The listing builds one solid part. Answer for the finished solid, in the listing's coordinates (mm). Face numbers are marked on the shaded views. A direction names the side the tool comes from. Round coordinates to 2 decimals unless told otherwise and drop trailing zeros. Order: outer loops, then holes, each group sorted by start corner. A loop starts at its lowest first (then second) coordinate and runs counter-clockwise, first axis right, second up. Notation, with made-up numbers: (1, 10.5) -> (9, 10.5) arc R20 ccw to (9, 34.5) -> close; hole circle Ø9 at (80.25, 6). An arc over 180 degrees is marked (long way). Answer in a Markdown table with one row per item. Add a question column.
```python
from build123d import *

# Parameters (mm, degrees)
SK_CBORE_R      = 5
BD_CBORE_DEPTH  = 5
SK_THREAD_R     = 2.5
BD_THREAD_DEPTH = 20
CF_CBORE_SIZE   = 0.5


with BuildPart() as part:
    # SK_CBORE → BD_CBORE (new body)
    with BuildSketch(Plane(origin=(0, 0, 0), x_dir=(0, 0, -1), z_dir=(0, 1, 0))):
        Circle(SK_CBORE_R)
    extrude(amount=BD_CBORE_DEPTH)

    # SK_THREAD → BD_THREAD (add)
    with BuildSketch(Plane.XZ):
        Circle(SK_THREAD_R)
    extrude(amount=BD_THREAD_DEPTH)

    # CF_CBORE
    cf_cbore_edges = [part.edges().sort_by_distance(p)[0] for p in [
        (0, 5, 5),
    ]]
    chamfer(cf_cbore_edges, length=CF_CBORE_SIZE)


solid = part.part
```
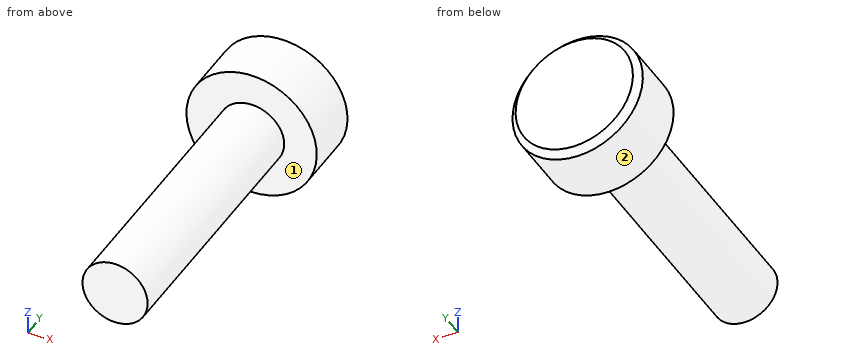
Item 1: Find the intervals of material crossed by probe 1 along Y at (x, z) = (3, 3); probe 2 along X at (y, z) = (-10, -1.5); probe 3 along Z at (x, y) = (2.5, 3.5), in increasing order. Write a range as [from, to].
Item 2: The part is cut by section A-A, the plane x = 0. Give the vertices of the cut face in (y, z), and give its area (3 significant figures).
Item 3: The part is cut by section C-C, the plane y = -4.5. Give the vertices of the cut face in (x, z), and give its area (3 significant figures).
Item 4: Flat-ended cylindrical pins translate along their axes: P1, Ø5, axis at x = -2.5, y = -9.5, coming from the +Z side; P2, Ø2, axis at y = -9.5, z = -1, coming from the +X side. Find the tip coordinate at first contact, or state that the pin passes through.
Item 5: A tool of negligible diameter and unlimited length cuts with its end or side. For the marked faces 1 and 2, from which of +Z, -Z, +X, -X, +Y, -Y can it reach the whole face along a straight path? Write none if from no direction.
Item 6: The part is cut by section B-B, the plane z = 0. Give the vertices of the cut face in (x, y).
Resolved:
| question | item | result |
|---|---|---|
| 1 | probe 1 | [0, 5] |
| 1 | probe 2 | [-2, 2] |
| 1 | probe 3 | [-4.33, 4.33] |
| 2 | outline | (-20, -2.5) -> (0, -2.5) -> (0, -5) -> (4.5, -5) -> (5, -4.5) -> (5, 4.5) -> (4.5, 5) -> (0, 5) -> (0, 2.5) -> (-20, 2.5) -> close |
| 2 | area | 150 mm2 |
| 3 | outline | circle Ø5 at (0, 0) |
| 3 | area | 19.6 mm2 |
| 4 | P1 | z = 2.5 |
| 4 | P2 | x = 2.5 |
| 5 | face 1 | -Y |
| 5 | face 2 | +Y, -Y |
| 6 | outline | (-5, 0) -> (-2.5, 0) -> (-2.5, -20) -> (2.5, -20) -> (2.5, 0) -> (5, 0) -> (5, 4.5) -> (4.5, 5) -> (-4.5, 5) -> (-5, 4.5) -> close |
